Could you check a few things on this model? Use its own coordinates, in mm. Face numbers are marked on the shaded views. A direction names the side the tool comes from. Give positions to 0.01 mm unless a question says otherwise; leave off trailing zeros. Write each loop counter-clockwise with the first axis right and the second up, starting at its lowest first coordinate (ties: lowest second). Pieces come first, ordered by that corner, then holes. Notation, with made-up numbers: (-13, 64.25) - (36, 64.25) arc R28 ccw to (36, 86.25) - close; hole circle Ø2 at (78.25, 62). An arc over 180 degrees is marked (long way). Answer as a JSON object with one key per item and string values. Group by question number.
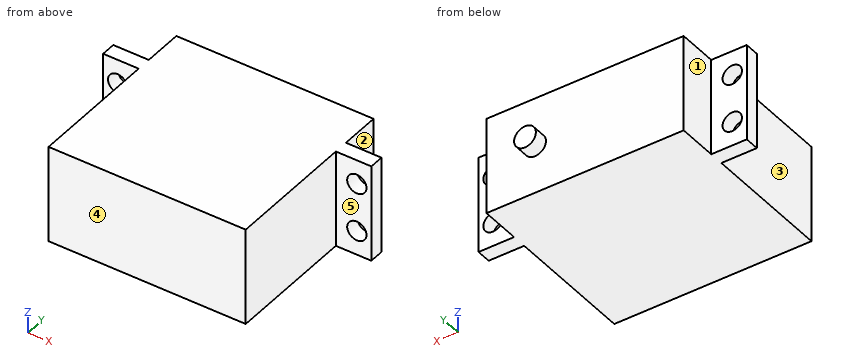
```python
from build123d import *

# Parameters (mm, degrees)
SKETCH1_W           = 40.8
SKETCH1_H           = 38
BOSS_EXTRUDE1_DEPTH = 20.1
SKETCH2_W           = 55.5
SKETCH2_H           = 3
BOSS_EXTRUDE2_DEPTH = 20.1
SKETCH3_R           = 2
CUT_EXTRUDE1_DEPTH  = 30.8
SKETCH4_R           = 2.25
BOSS_EXTRUDE3_DEPTH = 3


with BuildPart() as part:
    # Sketch1 → Boss-Extrude1 (new body)
    with BuildSketch(Plane.XY):
        with Locations((20.4, 19)):
            Rectangle(SKETCH1_W, SKETCH1_H)
    extrude(amount=BOSS_EXTRUDE1_DEPTH)

    # Sketch2 → Boss-Extrude2 (add)
    with BuildSketch(Plane.XY.offset(20.1)):
        with Locations((20.4, 28.3)):
            Rectangle(SKETCH2_W, SKETCH2_H)
    extrude(amount=-BOSS_EXTRUDE2_DEPTH)

    # Sketch3 → Cut-Extrude1 (cut, through all)
    with BuildSketch(Plane(origin=(0, 29.8, 0), x_dir=(1, 0, 0), z_dir=(0, 1, 0))):
        with Locations((-4.35, -5.05)):
            Circle(SKETCH3_R)
        with Locations((-4.35, -15.05)):
            Circle(SKETCH3_R)
        with Locations((45.15, -15.05)):
            Circle(SKETCH3_R)
        with Locations((45.15, -5.05)):
            Circle(SKETCH3_R)
    extrude(amount=-CUT_EXTRUDE1_DEPTH, mode=Mode.SUBTRACT)

    # Sketch4 → Boss-Extrude3 (add)
    with BuildSketch(Plane(origin=(0, 38, 0), x_dir=(1, 0, 0), z_dir=(0, 1, 0))):
        with Locations((30.75, -10.05)):
            Circle(SKETCH4_R)
    extrude(amount=BOSS_EXTRUDE3_DEPTH)


solid = part.part
```
(1) Will these pins go through, and if not, where does the flat tip stop? P1, Ø6, axis at x = -2, z = 14.5, coming from the +Y side; P2, Ø2, axis at y = 11, z = 3, coming from the +X side; P3, Ø2, axis at x = 44.5, z = 11.5, coming from the -Y side; P4, Ø2.5, axis at x = -4.35, z = 15.05, coming from the +Y side.
(2) For the marked faces 1, 2, 3, 4 and 5, which set-ups out of +Z, -Z, +X, -X, +Y, -Y let a thin tool reach every point of the face, with its end or its side?
(3) I want a section at C-C, the plane x = 30.75. Please give me the cut outline in (y, z), and give its area (3 significant figures).
(4) I want a section at B-B, the plane x = 45.15. Please give me the cut outline in (y, z), and give its area (3 significant figures).
(5) I want a section at D-D, the plane z = 6.25. Please give me the cut outline in (x, y), and give its area (3 significant figures).
(6) I need wall thicknesses on L1, parallel to X at y = 28.2, z = 5.05; L2, parallel to Z at x = -4.35, y = 27.8; L3, parallel to Z at x = -3, y = 28. Which ranges of each line are inside material? Lowest first, please.
(7) I want a section at A-A, the plane z = 15.05. Please give me the cut outline in (x, y).
Entries:
{
 "1": {"P1": "y = 38", "P2": "x = 40.8", "P3": "y = 26.8", "P4": "through"},
 "2": {"face 1": "+Z, -Z, -X, +Y", "face 2": "+Z, -Z, +X, +Y", "face 3": "+Z, -Z, -X, -Y", "face 4": "+Z, -Z, +X, -X, -Y", "face 5": "+Z, -Z, +X, -Y"},
 "3": {"outline": "(0, 0) - (38, 0) - (38, 7.8) - (41, 7.8) - (41, 12.3) - (38, 12.3) - (38, 20.1) - (0, 20.1) - close", "area": "777 mm^2"},
 "4": {"outline": "(26.8, 0) - (29.8, 0) - (29.8, 3.05) - (26.8, 3.05) - close; (26.8, 7.05) - (29.8, 7.05) - (29.8, 13.05) - (26.8, 13.05) - close; (26.8, 17.05) - (29.8, 17.05) - (29.8, 20.1) - (26.8, 20.1) - close", "area": "36.3 mm^2"},
 "5": {"outline": "(-7.35, 26.8) - (-5.95, 26.8) - (-5.95, 29.8) - (-7.35, 29.8) - close; (-2.75, 26.8) - (0, 26.8) - (0, 0) - (40.8, 0) - (40.8, 26.8) - (43.55, 26.8) - (43.55, 29.8) - (40.8, 29.8) - (40.8, 38) - (0, 38) - (0, 29.8) - (-2.75, 29.8) - close; (46.75, 26.8) - (48.15, 26.8) - (48.15, 29.8) - (46.75, 29.8) - close", "area": "1,580 mm^2"},
 "6": {"L1": "-7.35 to -6.35, -2.35 to 43.15, 47.15 to 48.15", "L2": "0 to 3.05, 7.05 to 13.05, 17.05 to 20.1", "L3": "0 to 3.57, 6.53 to 13.57, 16.53 to 20.1"},
 "7": {"outline": "(-7.35, 26.8) - (-6.35, 26.8) - (-6.35, 29.8) - (-7.35, 29.8) - close; (-2.35, 26.8) - (0, 26.8) - (0, 0) - (40.8, 0) - (40.8, 26.8) - (43.15, 26.8) - (43.15, 29.8) - (40.8, 29.8) - (40.8, 38) - (0, 38) - (0, 29.8) - (-2.35, 29.8) - close; (47.15, 26.8) - (48.15, 26.8) - (48.15, 29.8) - (47.15, 29.8) - close"}
}
